Part model, mm, in its own coordinate system. Face numbers are marked on the shaded views. A direction names the side the tool comes from. Round coordinates to 2 decimals unless told otherwise and drop trailing zeros. Write each loop counter-clockwise with the first axis right and the second up, starting at its lowest first coordinate (ties: lowest second). Pieces come first, ordered by that corner, then holes. Notation, with made-up numbers: M 61.5,-30.5 L 100.5,-30.5 A16 ccw 100.5,-25.5 Z; hole C 23,78.25 d9. An arc over 180 degrees is marked long. Use a Markdown table: item, result. Add a question column.
1) Slice it at A-A on x = 0.5. Write the cut outline in (y, z).
2) Slice it at B-B on y = 0. Write the cut outline in (x, z), plus the area to 3 significant figures.
3) Slice it at D-D on x = 2. Write the cut outline in (y, z).
4) Wall check: probe 1 along Y at (x, z) = (0, 2.25); probe 2 along X at (y, z) = (-4, 2.75); probe 3 along X at (y, z) = (-2, 8.5). Give the ranges that are in metal, low to high.
5) Slice it at C-C on z = 8.5. Write the cut outline in (x, y), plus the area to 3 significant figures.
6) Two-plate mould, pull along Y, no slides. Class the marked faces 4, 5, 6 and 7: released by +Y, released by -Y, zero draft, split by the parting line, or undercut.
7) Drop flat-ended pins along their axis: P1, Ø4, axis at y = -3, z = 8.5, coming from the -X side; P2, Ø6, axis at x = -1, y = 2, coming from the -Z side; P3, Ø5.5, axis at x = 0, y = 0, coming from the +Z side. Give the stop position or say it passes through.
8) Which spindle directions (+Z, -Z, +X, -X, +Y, -Y) get a long thin tool onto all of the face, cutting with end or side? Do the marked faces 1, 2 and 3. Say none if no direction does.
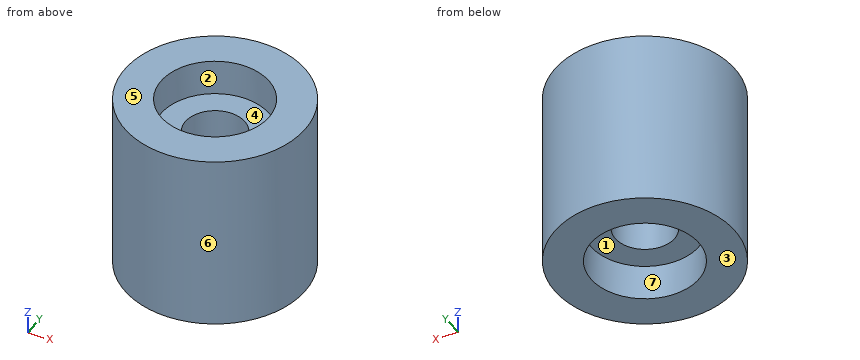
```python
from build123d import *

# Parameters (mm, degrees)
SKETCH1_R           = 5
BOSS_EXTRUDE1_DEPTH = 10
SKETCH2_R           = 3
CUT_EXTRUDE1_DEPTH  = 2
SKETCH3_R           = 1.65
CUT_EXTRUDE2_DEPTH  = 14
SKETCH4_R           = 3
CUT_EXTRUDE3_DEPTH  = 2


with BuildPart() as part:
    # Sketch1 → Boss-Extrude1 (new body)
    with BuildSketch(Plane.XY):
        Circle(SKETCH1_R)
    extrude(amount=BOSS_EXTRUDE1_DEPTH)

    # Sketch2 → Cut-Extrude1 (cut)
    with BuildSketch(Plane.XY):
        Circle(SKETCH2_R)
    extrude(amount=CUT_EXTRUDE1_DEPTH, mode=Mode.SUBTRACT)

    # Sketch3 → Cut-Extrude2 (cut)
    with BuildSketch(Plane.XY):
        Circle(SKETCH3_R)
    extrude(amount=CUT_EXTRUDE2_DEPTH, mode=Mode.SUBTRACT)

    # Sketch4 → Cut-Extrude3 (cut)
    with BuildSketch(Plane.XY.offset(10)):
        Circle(SKETCH4_R)
    extrude(amount=-CUT_EXTRUDE3_DEPTH, mode=Mode.SUBTRACT)


solid = part.part
```
Entries:
| question | item | result |
|---|---|---|
| 1 | outline | M -4.97,0 L -2.96,0 L -2.96,2 L -1.57,2 L -1.57,8 L -2.96,8 L -2.96,10 L -4.97,10 Z; M 1.57,2 L 2.96,2 L 2.96,0 L 4.97,0 L 4.97,10 L 2.96,10 L 2.96,8 L 1.57,8 Z |
| 2 | outline | M -5,0 L -3,0 L -3,2 L -1.65,2 L -1.65,8 L -3,8 L -3,10 L -5,10 Z; M 1.65,2 L 3,2 L 3,0 L 5,0 L 5,10 L 3,10 L 3,8 L 1.65,8 Z |
| 2 | area | 56.2 mm^2 |
| 3 | outline | M -4.58,0 L -2.24,0 L -2.24,2 L 2.24,2 L 2.24,0 L 4.58,0 L 4.58,10 L 2.24,10 L 2.24,8 L -2.24,8 L -2.24,10 L -4.58,10 Z |
| 4 | probe 1 | y = -5 to -1.65, 1.65 to 5 |
| 4 | probe 2 | x = -3 to 3 |
| 4 | probe 3 | x = -4.58 to -2.24, 2.24 to 4.58 |
| 5 | outline | C 0,0 d10; hole C 0,0 d6 |
| 5 | area | 50.3 mm^2 |
| 6 | face 4 | undercut |
| 6 | face 5 | zero draft |
| 6 | face 6 | split by the parting line |
| 6 | face 7 | undercut |
| 7 | P1 | stops at x = -4.9 |
| 7 | P2 | stops at z = 0 |
| 7 | P3 | stops at z = 8 |
| 8 | face 1 | -Z |
| 8 | face 2 | +Z |
| 8 | face 3 | -Z, +X, -X, +Y, -Y |
